from build123d import *

# Parameters (mm, degrees)
SKETCH1_R           = 14
BOSS_EXTRUDE1_DEPTH = 2
SKETCH2_R           = 14
SKETCH2_R_2         = 8
BOSS_EXTRUDE2_DEPTH = 7.5
SKETCH3_R           = 5
CUT_EXTRUDE1_DEPTH  = 2
SKETCH5_R           = 1.15
CUT_EXTRUDE2_DEPTH  = 22.960191256
SKETCH7_R           = 1.75
CUT_EXTRUDE3_DEPTH  = 7
SKETCH9_R           = 1.75
CUT_EXTRUDE4_DEPTH  = 7


with BuildPart() as part:
    # Sketch1 → Boss-Extrude1 (new body)
    with BuildSketch(Plane.XY):
        Circle(SKETCH1_R)
    extrude(amount=BOSS_EXTRUDE1_DEPTH)

    # Sketch2 → Boss-Extrude2 (add)
    with BuildSketch(Plane.XY.offset(2)):
        Circle(SKETCH2_R)
        Circle(SKETCH2_R_2, mode=Mode.SUBTRACT)
    extrude(amount=BOSS_EXTRUDE2_DEPTH)

    # Sketch3 → Cut-Extrude1 (cut)
    with BuildSketch(Plane(origin=(0, 0, 0), x_dir=(-1, 0, 0), z_dir=(0, 0, -1))):
        Circle(SKETCH3_R)
    extrude(amount=-CUT_EXTRUDE1_DEPTH, mode=Mode.SUBTRACT)

    # Sketch5 → Cut-Extrude2 (cut, through all)
    with BuildSketch(Plane.XY.offset(9.5)):
        with Locations((0, 10.85)):
            Circle(SKETCH5_R)
        with Locations((10.85, 0)):
            Circle(SKETCH5_R)
        with Locations((0, -10.85)):
            Circle(SKETCH5_R)
        with Locations((-10.85, 0)):
            Circle(SKETCH5_R)
    extrude(amount=-CUT_EXTRUDE2_DEPTH, mode=Mode.SUBTRACT)

    # Sketch7 → Cut-Extrude3 (cut)
    with BuildSketch(Plane(origin=(9.899494937, 9.899494937, 0), x_dir=(0.7071067811865489, -0.7071067811865461, 0), z_dir=(0.7071067811865461, 0.7071067811865489, 0))):
        with Locations(Location((0, -5.75, 0), (0, 0, 180))):
            Circle(SKETCH7_R)
    extrude(amount=-CUT_EXTRUDE3_DEPTH, mode=Mode.SUBTRACT)

    # Sketch9 → Cut-Extrude4 (cut)
    with BuildSketch(Plane(origin=(-9.899494937, 9.899494937, 0), x_dir=(0, 0, 1), z_dir=(-0.7071067811865489, 0.7071067811865462, 0))):
        with Locations(Location((5.75, 0, 0), (0, 0, 270))):
            Circle(SKETCH9_R)
    extrude(amount=-CUT_EXTRUDE4_DEPTH, mode=Mode.SUBTRACT)


solid = part.part
Design review of the part built by this model. Coordinates are the model's own, in mm. A direction names the side the tool comes from. Coordinates: 2 decimals unless noted, no trailing zeros. Order: outer loops, then holes, each group sorted by start corner. A loop starts at its lowest first (then second) coordinate and runs counter-clockwise, first axis right, second up. Notation, with made-up numbers: (-34.75, 85.25) -> (-6.75, 85.25) arc R19 cw to (-6.75, 118.25) -> close; hole circle Ø9 at (64.5, -2.75). An arc over 180 degrees is marked (long way). Use one line per item in the form item = value. Start each with the question number.
(1) Insertion check: pin 1 (13 mm diameter, centred on x = 0, y = 0, fed in from +Z); pin 2 (3 mm diameter, centred on x = -4, z = 5, fed in from -Y) (3 decimals); pin 3 (1.8 mm diameter, centred on x = -10.85, y = 0, fed in from -Z); pin 4 (4 mm diameter, centred on y = -3.5, z = 3.5, fed in from -X). Each pin has a flat end and moves straight along its axis. Give the tip position at first contact, or say it passes through.
(2) The part is to be moulded in two halves that separate along X. For faces 1 (the flat face through (0, -6, 0)), 2 (the cylindrical face through (9.7, 0.05, 4.82)), 3 (the cylindrical face through (6.5, -12.4, 4.7)), say which applies: +X half, -X half, draft (parallel to the pull), parting line (faces both ways), or undercut.
(3) Add section A-A on x = 0. State the section outline as (y, z) points, plus the area to 3 significant figures.
(4) Add section D-D on z = 8.5. State the section outline as (x, y) points, plus the area to 3 significant figures.
(5) For faces 4 (the flat face through (6, -6, 9.5)), 5 (the flat face through (-0.1, -5.2, 2)), list the 3-axis set-ups (+Z, -Z, +X, -X, +Y, -Y) from which the entire face can be reached by the end or side of a thin tool; tool diameter is ignored.
(6) For probe 1 along Y at (x, z) = (0, 2.75); probe 2 along Z at (x, y) = (1, 7.5); probe 3 along X at (y, z) = (-5.25, 4.5), list the stretches that pass through material, from the lowest coordinate up.
(7) Add section B-B on z = 6.75. State the section outline as (x, y) points, plus the area to 3 significant figures.
Answer block:
q1.pin_1 = 2
q1.pin_2 = -13.775
q1.pin_3 = through
q1.pin_4 = -13.92
q2.face_1 = draft
q2.face_2 = undercut
q2.face_3 = parting line
q3.outline = (-14, 0) -> (-12, 0) -> (-12, 9.5) -> (-14, 9.5) -> close; (-9.7, 0) -> (-5, 0) -> (-5, 2) -> (-8, 2) -> (-8, 9.5) -> (-9.7, 9.5) -> close; (5, 0) -> (9.7, 0) -> (9.7, 9.5) -> (8, 9.5) -> (8, 2) -> (5, 2) -> close; (12, 0) -> (14, 0) -> (14, 9.5) -> (12, 9.5) -> close
q3.area = 82.3 mm²
q4.outline = circle Ø28 at (0, 0); hole circle Ø2.3 at (-10.85, 0); hole circle Ø16 at (0, 0); hole circle Ø2.3 at (0, -10.85); hole circle Ø2.3 at (0, 10.85); hole circle Ø2.3 at (10.85, 0)
q4.area = 398 mm²
q5.face_4 = +Z, +X, -X, +Y, -Y
q5.face_5 = +Z
q6.probe_1 = -14 to -12, -9.7 to -8, 8 to 9.7, 12 to 14
q6.probe_2 = 0 to 2
q6.probe_3 = -12.98 to -6.04, 6.04 to 12.98
q7.outline = (-10.86, 8.83) arc R14 ccw (long way) to (10.86, 8.83) -> (6.58, 4.55) arc R8 cw (long way) to (-6.58, 4.55) -> close; (-8.83, 10.86) -> (-4.55, 6.58) arc R8 cw to (4.55, 6.58) -> (8.83, 10.86) arc R14 ccw to start; hole circle Ø2.3 at (-10.85, 0); hole circle Ø2.3 at (0, -10.85); hole circle Ø2.3 at (0, 10.85); hole circle Ø2.3 at (10.85, 0)
q7.area = 363 mm²
